Check sheet for the modelled part. Datum: model origin and axes. Units: mm. Face numbers are marked on the shaded views. A direction names the side the tool comes from. Give positions to 0.01 mm unless a question says otherwise; leave off trailing zeros. Order: outer loops, then holes, each group sorted by start corner. A loop starts at its lowest first (then second) coordinate and runs counter-clockwise, first axis right, second up.
from build123d import *

# Parameters (mm, degrees)
CROQUIS1_R              = 1.5
SALIENTE_EXTRUIR1_DEPTH = 10
CROQUIS2_W              = 8
CROQUIS2_H              = 7.5
CROQUIS2_W_2            = 9
CROQUIS2_H_2            = 8
CORTAR_EXTRUIR1_DEPTH   = 2.75
REDONDEO1_R             = 1


with BuildPart() as part:
    # Croquis1 → Saliente-Extruir1 (new, symmetric)
    with BuildSketch(Plane(origin=(0, 0, 0), x_dir=(0, 0, -1), z_dir=(1, 0, 0))):
        with BuildLine():
            Line((-15, -4), (15, -4))
            ThreePointArc((15, -4), (19, 0), (15, 4))
            Line((15, 4), (-13, 4))
            Line((-13, 4), (-13, 16))
            ThreePointArc((-13, 16), (-17, 20), (-21, 16))
            Line((-21, 16), (-21, 4))
            Line((-21, 4), (-43, 4))
            ThreePointArc((-43, 4), (-47, 0), (-43, -4))
            Line((-43, -4), (-15, -4))
        make_face()
        with Locations((15, 0)):
            Circle(CROQUIS1_R, mode=Mode.SUBTRACT)
        with Locations((-17, 16)):
            Circle(CROQUIS1_R, mode=Mode.SUBTRACT)
        with Locations((-15, 0)):
            Circle(CROQUIS1_R, mode=Mode.SUBTRACT)
        with Locations((-43, 0)):
            Circle(CROQUIS1_R, mode=Mode.SUBTRACT)
    extrude(amount=SALIENTE_EXTRUIR1_DEPTH, both=True)

    # Croquis2 → Cortar-Extruir1 (cut, symmetric)
    with BuildSketch(Plane(origin=(0, 0, 0), x_dir=(0, 0, -1), z_dir=(1, 0, 0))):
        with Locations((-17, 16.25)):
            Rectangle(CROQUIS2_W, CROQUIS2_H)
        with Locations((14.5, 0)):
            Rectangle(CROQUIS2_W_2, CROQUIS2_H_2)
        with Locations((-42.5, 0)):
            Rectangle(CROQUIS2_W_2, CROQUIS2_H_2)
    extrude(amount=CORTAR_EXTRUIR1_DEPTH, both=True, mode=Mode.SUBTRACT)

    # Redondeo1
    redondeo1_edges = [part.edges().sort_by_distance(p)[0] for p in [
        (2.75, 0, 38),
        (-2.75, 0, 38),
        (2.75, 0, -10),
        (-2.75, 0, -10),
    ]]
    fillet(redondeo1_edges, radius=REDONDEO1_R)


solid = part.part
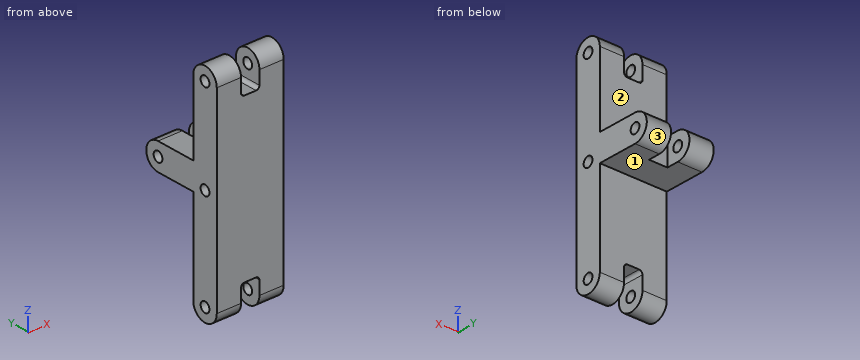
1) Depth check by flat-ended pin: pin 1 Ø6 at (x, z) = (-3, 32.5) entering from +Y; pin 2 Ø2.5 at (y, z) = (0, -15) entering from -X; pin 3 Ø6 at (x, y) = (0, 6.5) entering from +Z; pin 4 Ø4 at (x, y) = (5.5, 16) entering from -Z. Enter the tip coordinate at first touch or a pass-through.
Recorded:
pin 1: stops at y = 4
pin 2: passes through
pin 3: stops at z = 38
pin 4: stops at z = 13
2) Section check B-B, the plane y = 0. State how many separate pieces and enclosed holes the cut face has, then the cut area to 3 significant figures.
Recorded:
separate pieces: 6
enclosed holes: 0
area: 1,070 mm2
3) Section check D-D, the plane y = 6.5. Record the cut outline in (x, z), then the cut area to 3 significant figures.
Recorded:
outline: (-10, 13) - (10, 13) - (10, 21) - (-10, 21) - close
area: 160 mm2
4) Section check A-A, the plane x = -4.75. Record the cut outline in (y, z), then the cut area to 3 significant figures.
Recorded:
outline: (-4, -15) arc R4 ccw to (4, -15) - (4, 13) - (16, 13) arc R4 ccw to (16, 21) - (4, 21) - (4, 43) arc R4 ccw to (-4, 43) - close; hole circle Ø3 at (0, -15); hole circle Ø3 at (0, 15); hole circle Ø3 at (0, 43); hole circle Ø3 at (16, 17)
area: 607 mm2
5) Section check C-C, the plane z = 32.5. Record the cut outline in (x, y), then the cut area to 3 significant figures.
Recorded:
outline: (-10, -4) - (10, -4) - (10, 4) - (-10, 4) - close
area: 160 mm2
6) Set-up check for the marked faces 1, 2 and 3: record each of +Z, -Z, +X, -X, +Y, -Y from which the full face is reachable in a straight line by a thin tool's end or side.
Recorded:
face 1: -Z, +X, -X, +Y
face 2: +Z, +X, -X, +Y
face 3: +X, -X, +Y
7) Material ranges on L1, parallel to Z at x = -4.5, y = 16; L2, parallel to Y at x = -7.75, z = 17; L3, parallel to Y at x = -5.5, z = 32.5, recorded low to high.
Recorded:
L1: z = 13 to 15.5, 18.5 to 21
L2: y = -4 to 14.5, 17.5 to 20
L3: y = -4 to 4
